Autodesk Inventor part; units mm, degrees
ref_plane "Work Plane2" through (3.35, 0, 0) normal (0, 0, -1) x (1, 0, 0)
ref_plane "YZ Plane" through (0, 0, 0) normal (1, 0, 0) x (0, 1, 0)
ref_plane "XZ Plane" through (0, 0, 0) normal (0, 1, 0) x (-1, 0, 0)
sketch "Эскиз1" plane through (0, 0, 0) normal (0, 0, 1) x (1, 0, 0)
  line L0 (2.1, 0) -> (20, 0)
  line L1 (20, 0) -> (20, 1.5)
  line L2 (20, 1.5) -> (2.65, 1.5)
  line L3 (2.65, 1.5) -> (2.3433, 1.3466)
  line L4 (2.3433, 1.3466) -> (1.65, 1.3466)
  line L5 (0, 2.75) -> (0, 1.6)
  line L6 (0, 1.6) -> (1.6999, 0.7525)
  line L7 (1.6999, 0.7525) -> (2.1, 0)
  line L8 (-4, 0) -> (24, 0)
  line L9 (0, -0.55) -> (0, 3.3)
  line L10 (0, 2.75) -> (0.2466, 2.75)
  line L11 (0.2466, 2.75) -> (1.65, 1.3466)
  line L12 (2.65, 1.5) -> (1.4966, 1.5) construction
  dimension "d1" = 17.35
  dimension "d2" = 3
  dimension "d3" = 2.6933
  dimension "d4" = 3.2
  dimension "d5" = 26.5
  dimension "d6" = 62
  dimension "d7" = 2.1
  dimension "d8" = 0.3067
  dimension "d12" = 5.5
  dimension "d13" = 45
  dimension "d15" = 20
  dimension "d24" = 1.65
revolve "Базовый элемент" add sketch "Эскиз1" angle 360 about axis through (2.1, 0, 0) along (1, 0, 0) contours L7 L6 L5 L10 L11 L4 L3 L2 L1 L0
sketch "Эскиз2" plane through (0, 0, 0) normal (-1, 0, 0) x (0, 0, 1)
  line L0 (0, 1.6) -> (0, 0) construction
  line L1 (0, 0) -> (1.6, 0) construction
  arc A0 (0.48, 0) -> (0, 0.48) centre (0, 0) ccw construction
  arc A1 (0.56, 0) -> (0, 0.56) centre (0, 0) ccw construction
  arc A2 (1.5795, 0.255) -> (0.255, 1.5795) centre (0, 0) ccw
  line L2 (0, 0) -> (1.1314, 1.1314) construction
  line L3 (0.255, 1.5795) -> (0.2766, 0.4869)
  line L4 (1.5795, 0.255) -> (0.4869, 0.2766)
  arc A3 (0.255, 1.5795) -> (0, 1.6) centre (0, 0) ccw
  arc A4 (1.6, 0) -> (1.5795, 0.255) centre (0, 0) ccw
  line L5 (0, -3.85) -> (0, 3.85)
  line L6 (-3.85, 0) -> (3.85, 0)
  arc A5 (0.255, -1.5795) -> (1.5795, -0.255) centre (0, 0) ccw
  line L7 (0.255, -1.5795) -> (0.2766, -0.4869)
  line L8 (1.5795, -0.255) -> (0.4869, -0.2766)
  arc A6 (0, -1.6) -> (0.255, -1.5795) centre (0, 0) ccw
  arc A7 (1.5795, -0.255) -> (1.6, 0) centre (0, 0) ccw
  arc A8 (-0.255, 1.5795) -> (-1.5795, 0.255) centre (0, 0) ccw
  line L9 (-0.255, 1.5795) -> (-0.2766, 0.4869)
  line L10 (-1.5795, 0.255) -> (-0.4869, 0.2766)
  arc A9 (0, 1.6) -> (-0.255, 1.5795) centre (0, 0) ccw
  arc A10 (-1.5795, 0.255) -> (-1.6, 0) centre (0, 0) ccw
  arc A11 (-0.255, -1.5795) -> (0, -1.6) centre (0, 0) ccw
  arc A12 (-1.5795, -0.255) -> (-0.255, -1.5795) centre (0, 0) ccw
  arc A13 (-1.6, 0) -> (-1.5795, -0.255) centre (0, 0) ccw
  line L11 (-1.5795, -0.255) -> (-0.4869, -0.2766)
  line L12 (-0.255, -1.5795) -> (-0.2766, -0.4869)
  arc A14 (0.2766, 0.4869) -> (0.4869, 0.2766) centre (0.4912, 0.4912) ccw
  arc A15 (0.4869, -0.2766) -> (0.2766, -0.4869) centre (0.4912, -0.4912) ccw
  arc A16 (-0.4869, 0.2766) -> (-0.2766, 0.4869) centre (-0.4912, 0.4912) ccw
  arc A17 (-0.2766, -0.4869) -> (-0.4869, -0.2766) centre (-0.4912, -0.4912) ccw
  point P0 (1.1314, -1.1314)
  point P1 (-1.1314, 1.1314)
  point P2 (-1.1314, -1.1314)
  dimension "d17" = 0.96
  dimension "d18" = 1.12
  dimension "d19" = 3.2
  dimension "d20" = 45
  dimension "d21" = 0.255
extrude "Паз" add sketch "Эскиз2" against normal up to next draft 5 contours L4 A14 L3 A2 | A5 L7 A15 L8 | L9 A16 L10 A8 | A12 L11 A17 L12
fillet "Сопряжение1" radius 0.102 4 edges at (0, 1.6, 0) (0, 0, -1.6) (0, -1.6, 0) (0, 0, 1.6)
thread "Резьба"
chamfer "Фаска1" distance 0.3067 distance2 0.1534 1 edges at (20, -1.5, 0) measured on face at (20, 0.1367, 0.3027)
ref_plane "Work Plane2" through (3.35, 0, 0) normal (0, 0, -1) x (1, 0, 0)
equation "\"d1\" = GEL"
equation "\"d2\" = GD"
equation "\"d3\" = BDM"
equation "\"d4\" = SDM"
equation "\"d7\" = INTI"
equation "\"d8\" = GAL"
equation "\"d12\" = KOD"
equation "\"d13\" = 0.5 * SEWI"
equation "\"d15\" = NLG"
equation "\"d24\" = KOH"
equation "\"d17\" = 0.3 * SDM"
equation "\"d18\" = 0.35 * SDM"
equation "\"d19\" = SDM"
equation "\"d21\" = 0.5 * SBR"
equation "\"d23\" = 0.2 * SBR"
equation "\"d10\" = GEL"
equation "\"d25\" = -0.5 * SPD + 0.5 * GD"
equation "\"d26\" = 0.5 * GAL"
equation "\"NLG\" = 20"
equation "\"GEL\" = 17.35"
equation "\"GAL\" = 0.61345 * PTC"
equation "\"SPD\" = NND - 1.2269 * PTC"
equation "\"KOD\" = 5.5"
equation "\"KOH\" = 1.65"
equation "\"SBR\" = 0.51"
equation "\"INTI\" = 2.1"
equation "\"SDM\" = 3.2"
equation "\"GD\" = NND"
equation "\"BDM\" = NND - GAL"
equation "\"SEWI\" = 90deg"
equation "\"d9\" = SDM"
equation "\"GUL\" = 0.61345 * PTC"
equation "\"TOA\" = 30deg"
equation "\"EPV\" = 3.15"
equation "\"THREADDIA\" = 3"
equation "\"PTC\" = 0.5"
equation "\"NND\" = 3"
equation "\"GD1\" = THREADDIA - 1.2269 * PTC"
properties part number "ISO 7046-1 - M3 x 20 - 4.8 - H" material "Сталь"
Source: CAD feature listing. Evaluate the final solid. Frame: model axes, mm. A direction names the side the tool comes from. Coordinates: 2 decimals unless noted, no trailing zeros. Write each loop counter-clockwise with the first axis right and the second up, starting at its lowest first coordinate (ties: lowest second). Pieces come first, ordered by that corner, then holes. Notation, with made-up numbers: (-5, 64) -> (37, 64) arc R13 cw to (37, 76) -> close; hole circle Ø9 at (-7.75, -30). An arc over 180 degrees is marked (long way). Return JSON: item names as keys, results as strings. Group by question number.
1) Contact query for flat-ended pins moving along their axis: P1, Ø1, axis at x = 6.5, y = 0, coming from the +Z side; P2, Ø1, axis at x = 14.5, z = -1, coming from the -Y side. Output: stop coordinate, or through.
2) Set-up query: faces 1 (the face through (20, 0, 0)), 2 (the face through (11.13, -1.5, -0.07)), 3 (the face through (0.867, 0.003, -1.168)). Return all of +Z, -Z, +X, -X, +Y, -Y with unobstructed straight access to the full face (end or side cutting, diameter ignored); none if empty.
3) Mould query, pull axis Z, two halves, no side actions, for faces 4 (the face through (0.867, -0.003, 1.168)), 5 (the face through (1.992, -1.345, -0.059)), 6 (the face through (2.03, -0.1, -0.09)), 7 (the face through (0, 1, -1)). Classes: +Z half, -Z half, draft (parallel to the pull), parting line (faces both ways), or undercut.
4) Ray query, line 1 along Y through (x, z) = (3.75, 0.65); line 2 along Y through (x, z) = (17, -0.05); line 3 along X through (y, z) = (0.25, 2.5). Return the intervals inside material, ascending.
5) Section query A-A, the plane x = 13.25. Return loops of the section in (y, z).
From the geometry:
{
 "1": {"P1": "z = 1.5", "P2": "y = -1.41"},
 "2": {"face 1": "+Z, -Z, +X, +Y, -Y", "face 2": "+X", "face 3": "-X"},
 "3": {"face 4": "undercut", "face 5": "parting line", "face 6": "undercut", "face 7": "draft"},
 "4": {"line 1": "-1.35 to 1.35", "line 2": "-1.5 to 1.5", "line 3": "0 to 0.48"},
 "5": {"outline": "circle Ø3 at (0, 0)"}
}
